from build123d import *

# Parameters (mm, degrees)
TOP_PLATE_DIAMETER_R           = 73.025
TOP_PLATE_EXTRUDE_DEPTH        = 12.7
FUEL_PORT_CLEARANCE_DIAMETER_R = 12.7
FUEL_PORT_CLEARANCE_HOLE_DEPTH = 13.7
ASSEMBLY_BOLT_DIAMETER_R       = 2.97688
ASSEMBLY_BOLT_DEPTH            = 12.7
CIRPATTERN1_COUNT              = 18
LOX_PORT_REACH                 = 14.7
SKETCH7_R                      = 8.7122


with BuildPart() as part:
    # Top Plate Diameter → Top Plate Extrude (new body)
    with BuildSketch(Plane(origin=(0, 0, 0), x_dir=(1, 0, 0), z_dir=(0, 1, 0))):
        Circle(TOP_PLATE_DIAMETER_R)
    extrude(amount=TOP_PLATE_EXTRUDE_DEPTH)

    # Fuel Port Clearance Diameter → Fuel Port Clearance Hole (cut, through all)
    with BuildSketch(Plane(origin=(0, 12.7, 0), x_dir=(1, 0, 0), z_dir=(0, 1, 0))):
        Circle(FUEL_PORT_CLEARANCE_DIAMETER_R)
    extrude(amount=-FUEL_PORT_CLEARANCE_HOLE_DEPTH, mode=Mode.SUBTRACT)

    # Assembly Bolt Diameter → Assembly Bolt (cut)
    with BuildSketch(Plane(origin=(0, 12.7, 0), x_dir=(1, 0, 0), z_dir=(0, 1, 0))):
        with Locations((-65.016467368, 17.421109926)):
            Circle(ASSEMBLY_BOLT_DIAMETER_R)
    assembly_bolt = extrude(amount=-ASSEMBLY_BOLT_DEPTH, mode=Mode.SUBTRACT)

    # CirPattern1: Assembly Bolt ×18 about axis
    cirpattern1_axis = Axis((0, 0, 0), (0, 1, 0))
    for i in range(1, CIRPATTERN1_COUNT):
        add(assembly_bolt.rotate(cirpattern1_axis, i * 360 / CIRPATTERN1_COUNT), mode=Mode.SUBTRACT)

    # Sketch7 → LOX Port (cut, up to next)
    with BuildSketch(Plane(origin=(0, 12.7, 0), x_dir=(1, 0, 0), z_dir=(0, 1, 0)), mode=Mode.PRIVATE) as lox_port_sk1:
        with Locations((-30.226, 0)):
            Circle(SKETCH7_R)
    lox_port_tool1 = extrude(lox_port_sk1.sketch, amount=-LOX_PORT_REACH, mode=Mode.PRIVATE) & part.part
    add(lox_port_tool1.solids().sort_by_distance((-30.226, 12.7, 0))[0], mode=Mode.SUBTRACT)

    # Sketch9 → Cut-Revolve1 (revolve, cut)
    with BuildSketch(Plane.XY):
        with BuildLine():
            Line((-41.3385, 12.7), (-39.9923, 11.922771068))
            Line((-39.9923, 11.922771068), (-39.9923, 10.3124))
            ThreePointArc((-39.9923, 10.3124), (-39.953630803, 10.117996816), (-39.843510245, 9.953189755))
            Line((-39.843510245, 9.953189755), (-38.9382, 9.04787951))
            Line((-38.9382, 9.04787951), (-38.9382, 12.7))
            Line((-38.9382, 12.7), (-41.3385, 12.7))
        make_face()
    revolve(axis=Axis((-30.226, -7.468881995, 0), (0, 1, 0)), mode=Mode.SUBTRACT)


solid = part.part
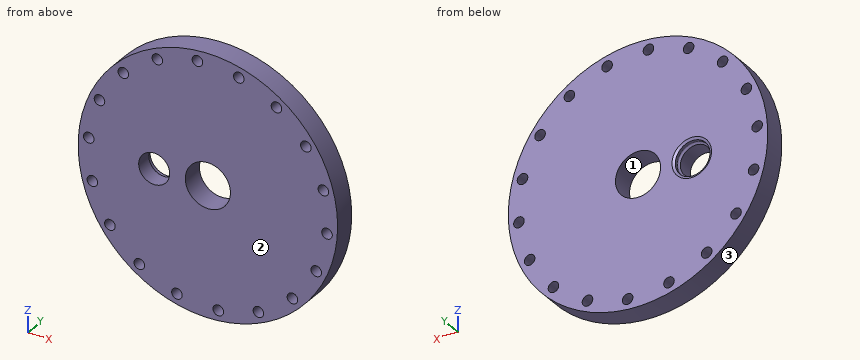
Input: part model. Units: mm. Frame: model coordinates. Face numbers are marked on the shaded views. Round coordinates to 2 decimals unless told otherwise and drop trailing zeros. Order: outer loops, then holes, each group sorted by start corner. A loop starts at its lowest first (then second) coordinate and runs counter-clockwise, first axis right, second up. Notation, with made-up numbers: (30, 37) - (56, 37) arc R22 ccw to (56, 47) - close; hole circle Ø1 at (-37.5, 59.25). An arc over 180 degrees is marked (long way). Answer as a JSON object with one key per item and string values. Group by question number.
(1) Cut plane C-C (z = -28.5). Return loops of the section in (x, y), then the cut area to 3 significant figures.
(2) Draft query along X for the marked faces 1, 2 and 3. Return one class per face: released by +X, released by -X, zero draft, split by the parting line, or undercut.
(3) Pin query (flat end, axial travel): P1, Ø4, axis at x = -3, y = 11, coming from the -Z side; P2, Ø3.5, axis at x = 17.42, z = 65.02, coming from the -Y side; P3, Ø2, axis at x = -44.5, y = 3, coming from the +Z side; P4, Ø1, axis at x = -38.5, y = 4.5, coming from the -Z side. Return the tip coordinate at first contact, or that it passes through.
(4) Cut plane A-A (z = 0). Count the separate pieces of the cut face and the enclosed holes in it, then the cut area to 3 significant figures.
(5) Material intervals for probe 1 along Z at (x, y) = (-36, 2.5); probe 2 along Z at (x, y) = (-29.5, 9.5); probe 3 along X at (y, z) = (8.75, 1), sorted ascending. Write a range as from..to.
(6) Cut plane B-B (x = 0). Return loops of the section in (y, z) (3 decimals), then the cut area to 3 significant figures.
Here are the results:
{
 "1": {"outline": "(-67.23, 0) - (58.03, 0) - (58.03, 12.7) - (-67.23, 12.7) - close; (63.98, 0) - (67.23, 0) - (67.23, 12.7) - (63.98, 12.7) - close", "area": "1,630 mm^2"},
 "2": {"face 1": "undercut", "face 2": "zero draft", "face 3": "split by the parting line"},
 "3": {"P1": "stops at z = -73.02", "P2": "passes through", "P3": "stops at z = 58.65", "P4": "stops at z = -62.36"},
 "4": {"separate pieces": "3", "enclosed holes": "0", "area": "1,300 mm^2"},
 "5": {"probe 1": "z = -63.53..-56.57, -53.7..-6.52, 6.52..63.53", "probe 2": "z = -66.8..-9.14, 9.14..58.22, 63.79..66.8", "probe 3": "x = -73.02..-38.88, -21.57..-12.66, 12.66..73.02"},
 "6": {"outline": "(0, -73.025) - (12.7, -73.025) - (12.7, -12.7) - (0, -12.7) - close; (0, 12.7) - (12.7, 12.7) - (12.7, 73.025) - (0, 73.025) - close", "area": "1,530 mm^2"}
}
